Autodesk Inventor part; units mm, degrees
ref_plane "YZ Plane" through (0, 0, 0) normal (1, 0, 0) x (0, 1, 0)
ref_plane "XZ Plane" through (0, 0, 0) normal (0, 1, 0) x (-1, 0, 0)
ref_plane "XY Plane" through (0, 0, 0) normal (0, 0, 1) x (1, 0, 0)
sketch "Szkic1" plane through (0, 0, 0) normal (0, 0, 1) x (1, 0, 0)
  line L0 (0, 0) -> (12, 0)
  line L1 (12, 0) -> (12, 21)
  line L2 (12, 21) -> (0, 21)
  line L3 (0, 21) -> (0, 0)
  dimension "d0" = 12
  dimension "d1" = 21
extrude "Wyciągnięcie proste1" add sketch "Szkic1" along normal blind 21
sketch "Szkic2" plane through (0, 0, 21) normal (0, 0, 1) x (1, 0, 0)
  line L0 (12, 0) -> (12, 21)
  line L1 (0, 17) -> (12, 17)
  line L2 (12, 17) -> (12, 14)
  line L3 (12, 14) -> (0, 14)
  line L4 (0, 14) -> (0, 17)
  line L5 (0, 17) -> (0, 14)
  line L6 (0, 21) -> (0, 0)
  dimension "d4" = 17
  dimension "d5" = 3
  dimension "d6" = 12
extrude "Wyciągnięcie proste2" add sketch "Szkic2" along normal blind 5
sketch "Szkic3" plane through (0, 0, 0) normal (0, 0, -1) x (-1, 0, 0)
  line L0 (0, 17) -> (0, 14)
  line L1 (-12, 14) -> (0, 14)
  line L2 (0, 14) -> (0, 17)
  line L3 (0, 17) -> (-12, 17)
  line L4 (0, 17) -> (-12, 17)
  line L5 (-12, 14) -> (-12, 17)
  line L6 (-12, 17) -> (-12, 14)
  point P0 (0, 0)
  point P1 (-12, 0)
extrude "Wyciągnięcie proste3" add sketch "Szkic3" along normal blind 5
sketch "Szkic4" plane through (0, 21, 0) normal (0, 1, 0) x (1, 0, 0)
  line L0 (12, -21) -> (0, -21)
  circle A0 centre (6, -16) radius 5
  point P0 (0, 0)
  dimension "d12" = 10
  dimension "d13" = 7.8102
extrude "Wyciągnięcie proste4" add sketch "Szkic4" along normal blind 5
sketch "Szkic5" plane through (6, 26, 16) normal (0, 1, 0) x (1, 0, 0)
  circle A0 centre (0, 0) radius 3.5
  point P0 (-6, 16)
  dimension "d16" = 7
extrude "Wyciągnięcie proste5" add sketch "Szkic5" along normal blind 4
sketch "Szkic6" plane through (6, 30, 16) normal (0, 1, 0) x (1, 0, 0)
  arc A0 (1.654, 14.1744) -> (-1.6556, 14.1022) centre (0, 14.1022) ccw
  line L0 (-1.6556, 14.1022) -> (-3.5, 0)
  circle A1 centre (0, 0) radius 3.5
  line L1 (1.654, 14.1744) -> (3.5266, 0)
  point P0 (-6, 16)
  point P1 (-3.3823, 0.9001)
  point P2 (3.4448, 0.6189)
  dimension "d19" = 1.6556
  dimension "d20" = 14.977
  dimension "d21" = 3.4962
  dimension "d22" = 3.4704
  dimension "d23" = 7.349
  dimension "d24" = 6.9673
  dimension "d25" = 3.2723
  dimension "d26" = 1.6493
extrude "Wyciągnięcie proste6" add sketch "Szkic6" against normal blind 1 contours L1 A1 L0 A0
properties part number "serwo"
The model under review builds one solid part; all positions refer to its coordinate system, in mm. A direction names the side the tool comes from. Round coordinates to 2 decimals unless told otherwise and drop trailing zeros. Write each loop counter-clockwise with the first axis right and the second up, starting at its lowest first coordinate (ties: lowest second). Pieces come first, ordered by that corner, then holes. Notation, with made-up numbers: M 32,-9 L 88,-9 A19 ccw 88,15 Z; hole C 10.5,-40 d3. An arc over 180 degrees is marked long. Use CSV: the item, a comma, the result in double quotes. Start each with the question number.
(1) Tool access review of faces 1 (the face through (6, 7, 0)), 2 (the face through (6, 17, 23)), 3 (the face through (3.493, 29.507, 8.406)): name each direction out of +Z, -Z, +X, -X, +Y, -Y from which nothing blocks a thin tool from reaching the whole face with its end or side.
(2) Clearance check with flat-ended pins moving along their axes: P1, Ø1.2, axis at x = 3.5, y = 18.5, coming from the +Z side; P2, Ø1.5, axis at y = 22.5, z = 3, coming from the +X side; P3, Ø5.5, axis at x = 7.5, z = -3, coming from the -Y side; P4, Ø5.5, axis at x = 3.5, z = -3, coming from the +Y side. State where each tip first meets the part, or that it passes through.
(3) We need section C-C, the plane y = 23. State the section outline as (x, z) points, then the cut area to 3 significant figures.
(4) The part is to be moulded in two halves that separate along Y. For faces 4 (the face through (0, 11, 10)), 5 (the face through (6, 29, 8)), 6 (the face through (5.54, 27.97, 19.47)), 7 (the face through (6, 14, 23)), say which applies: +Y half, -Y half, draft (parallel to the pull), parting line (faces both ways), or undercut.
(5) We need section D-D, the plane x = 5.25. State the section outline as (y, z) points.
(6) We need section A-A, the plane z = 16. State the section outline as (x, y) points.
(7) For line 1 along Y through (x, z) = (6.5, 8.5); line 2 along Y through (x, z) = (4.25, 11.5); line 3 along Y through (x, z) = (3, 11.5), list the stretches that pass through material, from the lowest coordinate up.
(8) We need section B-B, the plane z = 7.5. State the section outline as (x, y) points, then the cut area to 3 significant figures.
Findings:
1,face 1,"-Z, +X, -X, -Y"
1,face 2,"+Z, +X, -X, +Y"
1,face 3,"-Z, -X, +Y"
2,P1,"z = 21"
2,P2,"through"
2,P3,"y = 14"
2,P4,"y = 17"
3,outline,"C 6,16 d10"
3,area,"78.5 mm^2"
4,face 4,"draft"
4,face 5,"undercut"
4,face 6,"undercut"
4,face 7,"-Y half"
5,outline,"M 0,0 L 14,0 L 14,-5 L 17,-5 L 17,0 L 21,0 L 21,11.06 L 26,11.06 L 26,12.58 L 29,12.58 L 29,0.42 L 30,0.42 L 30,19.42 L 26,19.42 L 26,20.94 L 21,20.94 L 21,21 L 17,21 L 17,26 L 14,26 L 14,21 L 0,21 Z"
6,outline,"M 0,0 L 12,0 L 12,21 L 11,21 L 11,26 L 9.5,26 L 9.5,30 L 2.5,30 L 2.5,26 L 1,26 L 1,21 L 0,21 Z"
7,line 1,"0 to 21, 29 to 30"
7,line 2,"0 to 26, 29 to 30"
7,line 3,"0 to 21"
8,outline,"M 0,0 L 12,0 L 12,21 L 0,21 Z; M 3.61,29 L 8.4,29 L 8.4,30 L 3.61,30 Z"
8,area,"257 mm^2"
